Here's the drawing with two shaded views (mm, measured from the low corner). I have some questions. Coordinates: 2 decimals unless noted, no trailing zeros. Write each loop counter-clockwise with the first axis right and the second up, starting at its lowest first coordinate (ties: lowest second). Pieces come first, ordered by that corner, then holes.
Item 1: If I drill on probe 1 along Y at (x, z) = (29.5, 25); probe 2 along X at (y, z) = (21, 3); probe 3 along X at (y, z) = (18, 13), over which ranges is the centre line in solid material (lowest first)?
Item 2: I want a section at C-C on z = 27. Please give me the cut outline in (x, y), then the cut area to 3 significant figures.
Item 3: I want a section at A-A on z = 10. Please give me the cut outline in (x, y).
Item 4: I want a section at B-B on y = 9. Please give me the cut outline in (x, z) (1 decimal).
Item 5: For P1, Ø11.5, axis at x = 23.5, z = 14.5, coming from the -Y side; P2, Ø5, axis at y = 14, z = 6.5, coming from the +X side; P3, Ø12, axis at y = 26.5, z = 33, coming from the +X side, each with a flat end and sliding along its axis, tell me the tip position at first contact or that it passes through.
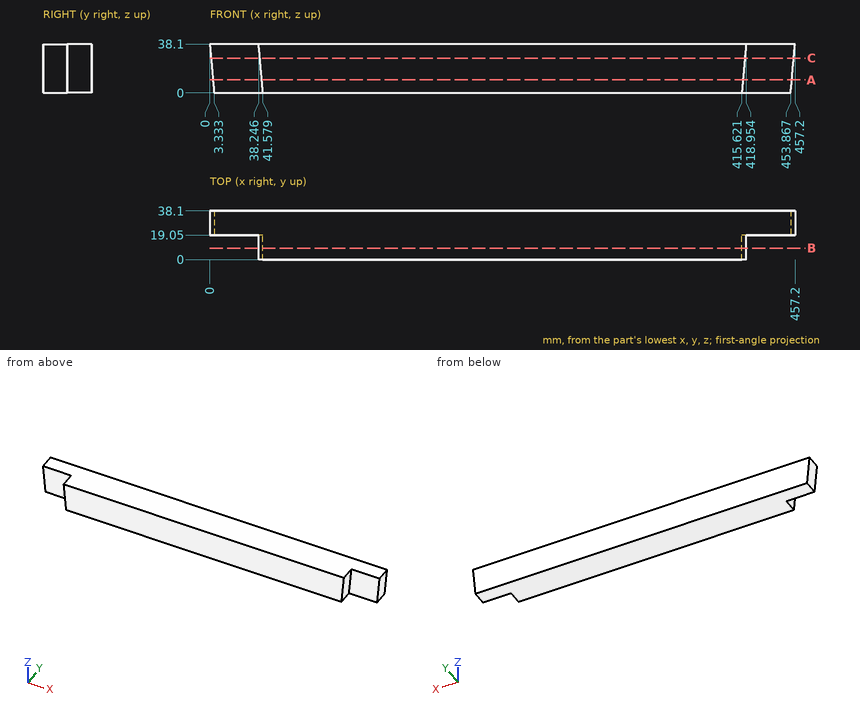
Response values:
1. probe 1: y = 19.05 to 38.1
1. probe 2: x = 3.07 to 454.13
1. probe 3: x = 40.44 to 416.76
2. outline: (0.97, 19.05) - (39.22, 19.05) - (39.22, 0) - (417.98, 0) - (417.98, 19.05) - (456.23, 19.05) - (456.23, 38.1) - (0.97, 38.1) - close
2. area: 15,900 mm2
3. outline: (2.46, 19.05) - (40.7, 19.05) - (40.7, 0) - (416.5, 0) - (416.5, 19.05) - (454.74, 19.05) - (454.74, 38.1) - (2.46, 38.1) - close
4. outline: (38.2, 38.1) - (41.6, 0) - (415.6, 0) - (419, 38.1) - close
5. P1: stops at y = 19.05
5. P2: stops at x = 416.41
5. P3: stops at x = 457.2
